from build123d import *

# Parameters (mm, degrees)
F0_W           = 755.396
F0_H           = 139.7
F1_DEPTH       = 5.08
F3_D           = 8.5
F3_CBORE_D     = 14
F3_CBORE_DEPTH = 8.5


with BuildPart() as f1:
    # F0 (on Top) → F1 (new body)
    with BuildSketch(Plane.XY):
        with Locations((378.988484, 69.85)):
            Rectangle(F0_W, F0_H)
    extrude(amount=F1_DEPTH)

    # F3 (through all)
    with Locations(Plane.XY.offset(5.08)):
        with Locations((13.990484, 127), (38.984084, 111.9886), (38.984084, 61.976), (53.995484, 46.9646), (53.995484, 21.971), (104.008084, 46.9646), (154.020684, 21.971), (154.020684, 46.9646), (204.033284, 46.9646), (254.045884, 21.971), (254.045884, 46.9646), (304.058484, 46.9646), (354.071084, 46.9646), (354.071084, 21.971), (404.083684, 21.971), (404.083684, 46.9646), (454.096284, 46.9646), (504.108884, 21.971), (504.108884, 46.9646), (554.121484, 46.9646), (604.134084, 46.9646), (604.134084, 21.971), (743.986484, 127), (718.992884, 111.9886), (718.992884, 61.976), (704.159284, 46.9646), (704.159284, 21.971), (654.146684, 46.9646)):
            CounterBoreHole(F3_D / 2, F3_CBORE_D / 2, F3_CBORE_DEPTH)


solid = f1.part
The listing builds one solid part. Answer for the finished solid, in the listing's coordinates (mm). Coordinates: 2 decimals unless noted, no trailing zeros. Loops run counter-clockwise (first coordinate to the right, second up) from the corner with the lowest first, then second, coordinate; pieces in that order, holes last.
1) Find section B-B on z = 3. Give the number of separate pieces and of enclosed holes in the cut face, then the cut area to 3 significant figures.
2) Find section A-A on y = 127. Write down the section's boundary in (x, z), then the cut area to 3 significant figures.
3) A flat-ended cylindrical pin translates along its axis: pin 1 Ø12.5 at (x, y) = (718.99, 61.98) entering from -Z. Find the tip coordinate at first contact, or state that the pin passes through.
4) Find the intervals of material crossed by L1, parallel to X at y = 130.5, z = 2.3; L2, parallel to X at y = 55.5, z = 4.7; L3, parallel to Y at x = 352, z = 4, in increasing order.
5) Determine the mould class of faces 1 (the face through (410.76, 49.07, 2.58)), 2 (the face through (374, 71, 0)) for opening direction Y: pulls with the +Y half, pulls with the -Y half, needs draft (parallel to the pull), parting line crosses it, or undercut.
Values:
1. separate pieces: 1
1. enclosed holes: 28
1. area: 101,000 mm2
2. outline: (1.29, 0) - (6.99, 0) - (6.99, 5.08) - (1.29, 5.08) - close; (20.99, 0) - (736.99, 0) - (736.99, 5.08) - (20.99, 5.08) - close; (750.99, 0) - (756.69, 0) - (756.69, 5.08) - (750.99, 5.08) - close
2. area: 3,700 mm2
3. pin 1: passes through
4. L1: x = 1.29 to 7.93, 20.05 to 737.92, 750.05 to 756.69
4. L2: x = 1.29 to 36.33, 41.64 to 716.34, 721.65 to 756.69
4. L3: y = 0 to 15.28, 28.66 to 40.28, 53.65 to 139.7
5. face 1: undercut
5. face 2: needs draft
